CAD build for the part. Positions are in the model's coordinates, mm. A direction names the side the tool comes from. Coordinates: 2 decimals unless noted, no trailing zeros. Loops run counter-clockwise (first coordinate to the right, second up) from the corner with the lowest first, then second, coordinate; pieces in that order, holes last. Notation, with made-up numbers: (48, 45.25) -> (65, 45.25) arc R32 ccw to (65, 76.25) -> close; hole circle Ø7 at (82.5, 31.5). An arc over 180 degrees is marked (long way). Write item = value, one per line. Start each with the question number.
(1) Tool access for faces 1 (the face through (-1, -41, 48.58)), 2 (the face through (-8, -5.205, 13)), 3 (the face through (-1, -45, 27.6)): list every direction of +Z, -Z, +X, -X, +Y, -Y with a clear straight run to the whole face (end or side of a thin tool).
(2) Flat gauge pins, fed straight in: P1, Ø21, axis at y = 1.86, z = 46.03, coming from the +X side; P2, Ø8, axis at y = -10, z = 44.5, coming from the +X side; P3, Ø8, axis at x = -3.5, z = 59, coming from the -Y side; P4, Ø4, axis at y = -49.19, z = 69.31, coming from the +X side. Where does each tip first touch, or does it go through?
(3) Band-saw the part on A-A (y = -44.5). Write the cut outline in (x, z).
(4) Band-saw the part on C-C (z = 46.03). Write the cut outline in (x, y), and give its area (3 significant figures).
(5) Band-saw the part on B-B (x = 8). Count the separate pieces of the cut face and the enclosed holes in it, and give its area (3 significant figures).
(6) Drill centre lines: line 1 (Y direction, x = 5, z = 66); line 2 (Z direction, x = -7.75, y = -20); line 3 (Y direction, x = 2.5, z = 18.5). Where is each one in solid material? Low to high. Write a range as from..to.
(7) Pull direction Z, two halves, no side cores. Call faces 4 (the face through (-8, 6.495, 62)), 5 (the face through (-10, -4.355, 33)): +Z half, -Z half, draft (parallel to the pull), parting line (faces both ways), or undercut.
```python
from build123d import *

# Parameters (mm, degrees)
PROFILEEXTRUDE_DEPTH    = 73.76
HOSEWINDOW_W            = 16.29
HOSEWINDOW_H            = 26.5
HOSEWINDOWCUT_DEPTH     = 23.11
CAGESCREWS_R            = 2.4
CAGESCREWSCUT_DEPTH     = 23.11
AXLEHOLECUT_DEPTH       = 23.11
SETSCREWHOLES_R         = 1.539432213
SETSCREWHOLES_R_2       = 1.628953018
SETSCREWHOLESCUT_DEPTH  = 23.11
VELOCITYWINDOW_W        = 12.61
VELOCITYWINDOW_H        = 22.29
VELOCITYWINDOWCUT_DEPTH = 23.11
FILLET3_R               = 7
TRIGGERRACKSLOTCUT_W    = 6.5
TRIGGERRACKSLOTCUT_H    = 6.5
RACKSLOTCUT_DEPTH       = 23.11
FILLET4_R               = 1


with BuildPart() as part:
    # Profile → ProfileExtrude (new body)
    with BuildSketch(Plane.XY):
        with BuildLine():
            Line((9.301269376, -54.194713793), (9.301269376, -29.194713793))
            Line((9.301269376, -29.194713793), (-0.848730624, -29.194713793))
            Line((-0.848730624, -29.194713793), (-0.848730624, -13.196583793))
            ThreePointArc((-0.848730624, -13.196583793), (-4.204324299, -9.619560571), (-6.340730624, -5.204713793))
            Line((-6.340730624, -5.204713793), (-8.928730624, -5.204713793))
            Line((-8.928730624, -5.204713793), (-8.928730624, 6.495286207))
            Line((-8.928730624, 6.495286207), (-6.509650624, 6.495286207))
            ThreePointArc((-6.509650624, 6.495286207), (-4.210311879, 9.168674207), (-1.388730624, 11.283536207))
            Line((-1.388730624, 11.283536207), (-1.388730624, 21.845286207))
            Line((-1.388730624, 21.845286207), (10.261269376, 21.845286207))
            Line((10.261269376, 21.845286207), (10.261269376, 31.845286207))
            Line((10.261269376, 31.845286207), (-11.848730624, 31.845286207))
            Line((-11.848730624, 31.845286207), (-11.848730624, -54.194713793))
            Line((-11.848730624, -54.194713793), (9.301269376, -54.194713793))
        make_face()
    extrude(amount=PROFILEEXTRUDE_DEPTH)

    # HoseWindow → HoseWindowCut (cut, through all)
    with BuildSketch(Plane.ZY.offset(11.848730624)):
        with Locations((56.725, -40.944713793)):
            Rectangle(HOSEWINDOW_W, HOSEWINDOW_H)
    extrude(amount=-HOSEWINDOWCUT_DEPTH, mode=Mode.SUBTRACT)

    # CageScrews → CageScrewsCut (cut, through all)
    with BuildSketch(Plane.ZY.offset(11.848730624)):
        with Locations((7.5, 26.845286207)):
            Circle(CAGESCREWS_R)
        with Locations((66.26, 26.845286207)):
            Circle(CAGESCREWS_R)
        with Locations((7.5, -49.194713793)):
            Circle(CAGESCREWS_R)
        with Locations((69.31, -49.194713793)):
            Circle(CAGESCREWS_R)
    extrude(amount=-CAGESCREWSCUT_DEPTH, mode=Mode.SUBTRACT)

    # AxleHole → AxleHoleCut (cut, through all)
    with BuildSketch(Plane.ZY.offset(11.848730624)):
        with BuildLine():
            Line((47.361, 8.359497151), (47.361, 6.740497151))
            Line((47.361, 6.740497151), (44.699, 6.740497151))
            Line((44.699, 6.740497151), (44.699, 8.359497151))
            ThreePointArc((44.699, 8.359497151), (46.03, -4.783713793), (47.361, 8.359497151))
        make_face()
    extrude(amount=-AXLEHOLECUT_DEPTH, mode=Mode.SUBTRACT)

    # SetScrewHoles → SetScrewHolesCut (cut, through all)
    with BuildSketch(Plane.ZY.offset(11.848730624)):
        with Locations((6.03, 1.855286207)):
            Circle(SETSCREWHOLES_R)
        with Locations((68.03, 1.855286207)):
            Circle(SETSCREWHOLES_R_2)
    extrude(amount=-SETSCREWHOLESCUT_DEPTH, mode=Mode.SUBTRACT)

    # VelocityWindow → VelocityWindowCut (cut, through all)
    with BuildSketch(Plane.ZY.offset(11.848730624)):
        with Locations((32.655, -15.499713793)):
            Rectangle(VELOCITYWINDOW_W, VELOCITYWINDOW_H)
    extrude(amount=-VELOCITYWINDOWCUT_DEPTH, mode=Mode.SUBTRACT)

    # Fillet3
    fillet3_edges = [part.edges().sort_by_distance(p)[0] for p in [
        (-11.848730624, -26.644713793, 32.655),
    ]]
    fillet(fillet3_edges, radius=FILLET3_R)

    # TriggerRackSlotCut → RackSlotCut (cut, through all)
    with BuildSketch(Plane.ZY.offset(11.848730624)):
        with Locations((18.25, -44.594713793)):
            Rectangle(TRIGGERRACKSLOTCUT_W, TRIGGERRACKSLOTCUT_H)
        with Locations((30.85, -44.594713793)):
            Rectangle(TRIGGERRACKSLOTCUT_W, TRIGGERRACKSLOTCUT_H)
        with Locations((5.65, -31.894713793)):
            Rectangle(TRIGGERRACKSLOTCUT_W, TRIGGERRACKSLOTCUT_H)
        with Locations((18.25, -31.894713793)):
            Rectangle(TRIGGERRACKSLOTCUT_W, TRIGGERRACKSLOTCUT_H)
        with Locations((5.65, -16.894713793)):
            Rectangle(TRIGGERRACKSLOTCUT_W, TRIGGERRACKSLOTCUT_H)
        with Locations((18.25, -16.894713793)):
            Rectangle(TRIGGERRACKSLOTCUT_W, TRIGGERRACKSLOTCUT_H)
    extrude(amount=-RACKSLOTCUT_DEPTH, mode=Mode.SUBTRACT)

    # Fillet4
    fillet4_edges = [part.edges().sort_by_distance(p)[0] for p in [
        (-11.848730624, -11.174713793, 73.76),
        (-11.848730624, -18.999713793, 26.35),
        (-11.848730624, -18.999713793, 38.96),
        (-11.848730624, -4.354713793, 32.655),
        (-11.848730624, -44.594713793, 15),
        (-11.848730624, -47.844713793, 18.25),
        (-11.848730624, -44.594713793, 21.5),
        (-11.848730624, -41.344713793, 18.25),
        (-11.848730624, -11.174713793, 0),
        (-11.848730624, -44.594713793, 27.6),
        (-11.848730624, -47.844713793, 30.85),
        (-11.848730624, -44.594713793, 34.1),
        (-11.848730624, -41.344713793, 30.85),
        (-11.848730624, -31.894713793, 2.4),
        (-11.848730624, -35.144713793, 5.65),
        (-11.848730624, -31.894713793, 8.9),
        (-11.848730624, -28.644713793, 5.65),
        (-11.848730624, -31.894713793, 15),
        (-11.848730624, -35.144713793, 18.25),
        (-11.848730624, -31.894713793, 21.5),
        (-11.848730624, -28.644713793, 18.25),
        (-11.848730624, -54.194713793, 69.315),
        (-11.848730624, 31.845286207, 36.88),
        (-11.848730624, -16.894713793, 2.4),
        (-11.848730624, -20.144713793, 5.65),
        (-11.848730624, -16.894713793, 8.9),
        (-11.848730624, -13.644713793, 5.65),
        (-11.848730624, -16.894713793, 15),
        (-11.848730624, -20.144713793, 18.25),
        (-11.848730624, -16.894713793, 21.5),
        (-11.848730624, -13.644713793, 18.25),
        (-11.848730624, -54.194713793, 24.29),
        (-11.848730624, -40.944713793, 64.87),
        (-11.848730624, -27.694713793, 56.725),
        (-11.848730624, -40.944713793, 48.58),
    ]]
    fillet(fillet4_edges, radius=FILLET4_R)


solid = part.part
```
Findings below:
q1.face_1 = +X, -X, -Y
q1.face_2 = +Z, -Z, +X
q1.face_3 = +X, -X
q2.P1 = -1.39
q2.P2 = -0.85
q2.P3 = -27.69
q2.P4 = through
q3.outline = (-11.85, 1) arc R1 ccw to (-10.85, 0) -> (9.3, 0) -> (9.3, 15) -> (-10.85, 15) arc R1 ccw to (-11.85, 14) -> close; (-11.85, 22.5) arc R1 ccw to (-10.85, 21.5) -> (9.3, 21.5) -> (9.3, 27.6) -> (-10.85, 27.6) arc R1 ccw to (-11.85, 26.6) -> close; (-11.85, 35.1) arc R1 ccw to (-10.85, 34.1) -> (9.3, 34.1) -> (9.3, 48.58) -> (-10.85, 48.58) arc R1 ccw to (-11.85, 47.58) -> close; (-11.85, 65.87) arc R1 ccw to (-10.85, 64.87) -> (9.3, 64.87) -> (9.3, 73.76) -> (-10.85, 73.76) arc R1 ccw to (-11.85, 72.76) -> close
q4.outline = (-11.85, -53.19) arc R1 ccw to (-10.85, -54.19) -> (9.3, -54.19) -> (9.3, -29.19) -> (-0.85, -29.19) -> (-0.85, -13.2) arc R16.26 cw to (-6.34, -5.2) -> (-8.93, -5.2) -> (-8.93, -4.78) -> (-11.85, -4.78) -> close; (-11.85, 6.74) -> (-6.34, 6.74) arc R16.26 cw to (-1.39, 11.28) -> (-1.39, 21.85) -> (10.26, 21.85) -> (10.26, 31.85) -> (-10.85, 31.85) arc R1 ccw to (-11.85, 30.85) -> close
q4.area = 1,130 mm²
q5.separate_pieces = 3
q5.enclosed_holes = 6
q5.area = 1,940 mm²
q6.line_1 = -54.19..-29.19, 21.85..24.46, 29.23..31.85
q6.line_2 = 0..2.4, 8.9..15, 21.5..26.35, 38.96..73.76
q6.line_3 = -54.19..-47.84, -41.34..-35.14, 21.85..31.85
q7.face_4 = draft
q7.face_5 = undercut
